Read the model definition and answer for the solid it produces. Units are mm, in the model's axes. Face numbers are marked on the shaded views. A direction names the side the tool comes from. Coordinates: 2 decimals unless noted, no trailing zeros. Order: outer loops, then holes, each group sorted by start corner. A loop starts at its lowest first (then second) coordinate and runs counter-clockwise, first axis right, second up. Notation, with made-up numbers: (-8.75, 4) - (25.25, 4) arc R23 ccw to (25.25, 19) - close; hole circle Ø8 at (-3, 46.5). An arc over 180 degrees is marked (long way). Use one line per item in the form item = value.
```python
from build123d import *

# Parameters (mm, degrees)
BOSS_EXTRUDE1_DEPTH = 10
CHAMFER4_SIZE       = 1
CHAMFER4_SIZE2      = 0.577350269
FILLET3_R           = 0.5
SKETCH3_R           = 2
SKETCH3_R_2         = 1.75
BOSS_EXTRUDE3_DEPTH = 2.5


with BuildPart() as part:
    # Sketch1 → Boss-Extrude1 (new body)
    with BuildSketch(Plane(origin=(0, 0, 0), x_dir=(-1, 0, 0), z_dir=(0, 1, 0))):
        Polygon((0, 1.5), (0, 1.75), (1.5, 1.75), (1.5, 6.75), (4.5, 6.75), (4.5, 1.75), (6, 1.75), (6, 1.5), align=None)
    extrude(amount=BOSS_EXTRUDE1_DEPTH)

    # Chamfer4
    chamfer4_edges = [part.edges().sort_by_distance(p)[0] for p in [
        (-1.5, 5, 6.75),
        (-4.5, 5, 6.75),
        (-3, 10, 6.75),
        (-3, 0, 6.75),
    ]]
    chamfer4_side = [part.faces().sort_by_distance(p)[0] for p in [
        (-3, 5, 6.75),
    ]]
    chamfer(chamfer4_edges, length=CHAMFER4_SIZE, length2=CHAMFER4_SIZE2, reference=chamfer4_side[0])

    # Fillet3
    fillet3_edges = [part.edges().sort_by_distance(p)[0] for p in [
        (-4.5, 5, 6.172649731),
        (-3, 10, 6.172649731),
        (-1.5, 5, 6.172649731),
        (-3, 0, 6.172649731),
    ]]
    fillet(fillet3_edges, radius=FILLET3_R)

    # Sketch3 → Boss-Extrude3 (add)
    with BuildSketch(Plane(origin=(0, 0, 1.5), x_dir=(1, 0, 0), z_dir=(0, 0, -1))):
        with Locations((-3, -5)):
            Circle(SKETCH3_R)
        with Locations(Location((-3, -5, 0), (0, 0, 180))):
            Circle(SKETCH3_R_2, mode=Mode.SUBTRACT)
    extrude(amount=BOSS_EXTRUDE3_DEPTH)


solid = part.part
```
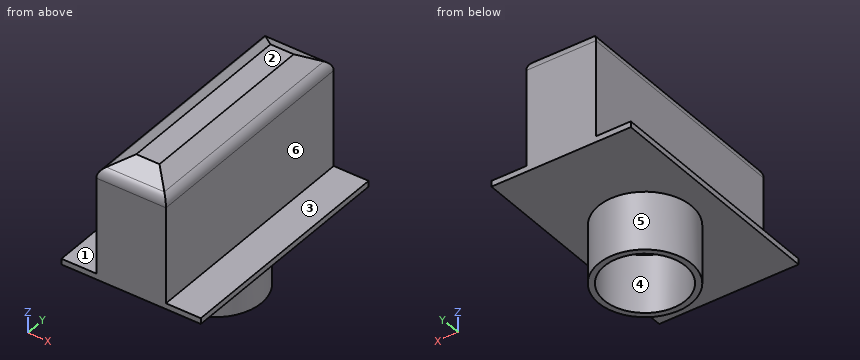
(1) Straight lines are drawn through the part: L1, parallel to Y at x = -3, z = -0.3; L2, parallel to X at y = 5, z = 2.25; L3, parallel to Z at x = -0.65, y = 4.25. For each, find the intervals that lie inside material, in ascending order.
Answer list:
L1 = 3 to 3.25, 6.75 to 7
L2 = -4.5 to -1.5
L3 = 1.5 to 1.75
(2) Section C-C, the plane z = 3 is taken. Write down the section's boundary in (x, y), then the cut area to 3 significant figures.
Answer list:
outline = (-4.5, 0) - (-1.5, 0) - (-1.5, 10) - (-4.5, 10) - close
area = 30.0 mm2
(3) The mould has two halves that part along X. Classify the marked faces 4, 5 and 6: +X half, -X half, draft (parallel to the pull), parting line (faces both ways), or undercut.
Answer list:
face_4 = undercut
face_5 = parting line
face_6 = +X half
(4) Section A-A, the plane x = -3 is taken. Write down the section's boundary in (y, z).
Answer list:
outline = (0, 1.5) - (3, 1.5) - (3, -1) - (3.25, -1) - (3.25, 1.5) - (6.75, 1.5) - (6.75, -1) - (7, -1) - (7, 1.5) - (10, 1.5) - (10, 5.88) arc R0.5 ccw to (9.75, 6.32) - (9, 6.75) - (1, 6.75) - (0.25, 6.32) arc R0.5 ccw to (0, 5.88) - close
(5) Given pin 1 Ø1.5 at (y, z) = (6.5, 5) entering from -X; pin 2 Ø1.5 at (x, z) = (-5, 0.5) entering from +Y; pin 3 Ø1 at (x, y) = (-3, 5.5) entering from -Z, each flat-ended and moving along its own axis, determine where each tip first touches the part or whether it passes through.
Answer list:
pin_1 = -4.5
pin_2 = 6.56
pin_3 = 1.5
(6) Section B-B, the plane y = 5 is taken. Write down the section's boundary in (x, z).
Answer list:
outline = (-6, 1.5) - (-5, 1.5) - (-5, -1) - (-4.75, -1) - (-4.75, 1.5) - (-1.25, 1.5) - (-1.25, -1) - (-1, -1) - (-1, 1.5) - (0, 1.5) - (0, 1.75) - (-1.5, 1.75) - (-1.5, 5.88) arc R0.5 ccw to (-1.75, 6.32) - (-2.5, 6.75) - (-3.5, 6.75) - (-4.25, 6.32) arc R0.5 ccw to (-4.5, 5.88) - (-4.5, 1.75) - (-6, 1.75) - close
(7) Section D-D, the plane y = 7.25 is taken. Write down the section's boundary in (x, z).
Answer list:
outline = (-6, 1.5) - (0, 1.5) - (0, 1.75) - (-1.5, 1.75) - (-1.5, 5.88) arc R0.5 ccw to (-1.75, 6.32) - (-2.5, 6.75) - (-3.5, 6.75) - (-4.25, 6.32) arc R0.5 ccw to (-4.5, 5.88) - (-4.5, 1.75) - (-6, 1.75) - close
(8) Which of the six approach directions +Z, -Z, +X, -X, +Y, -Y give full straight-line access (tool end or side, diameter ignored) to the marked faces 1, 2 and 3?
Answer list:
face_1 = +Z, -X, +Y, -Y
face_2 = +Z, +X, -X, +Y, -Y
face_3 = +Z, +X, +Y, -Y
